The model under review builds one solid part; all positions refer to its coordinate system, in mm. Face numbers are marked on the shaded views. A direction names the side the tool comes from. Coordinates: 2 decimals unless noted, no trailing zeros. Write each loop counter-clockwise with the first axis right and the second up, starting at its lowest first coordinate (ties: lowest second). Pieces come first, ordered by that corner, then holes. Notation, with made-up numbers: (-3.5, 72.5) - (3.5, 72.5) arc R31 ccw to (3.5, 110.5) - close; hole circle Ø11 at (29, 18). An arc over 180 degrees is marked (long way). Return JSON: item names as keys, results as strings. Group by question number.
(1) We need section B-B on z = 21.25. State the section outline as (x, y) points, then the cut area to 3 significant figures.
(2) Tool access review of the marked faces 1, 2 and 3: name each direction out of +Z, -Z, +X, -X, +Y, -Y from which nothing blocks a thin tool from reaching the whole face with its end or side.
(3) For pin 1 Ø5 at (x, z) = (68.18, 6.66) entering from +Y; pin 2 Ø12 at (x, z) = (44.5, 17) entering from +Y; pin 3 Ø3 at (y, z) = (25.5, 7) entering from +X; pin 4 Ø3 at (x, z) = (50.82, 17.34) entering from +Y, all flat-tipped, find the tip position at first contact; note any pin that passes through.
(4) We need section C-C on y = 15.5. State the section outline as (x, z) points.
(5) To check wall thickness, follow L1, parallel to Y at x = 37, z = 20; L2, parallel to Z at x = 20, y = 3.95; L3, parallel to Y at x = 52.5, z = 8.75. State the ranges of each line that lie inside material, in increasing order. Write a range as from..to.
(6) We need section A-A on x = 20. State the section outline as (y, z) points.
(7) Draft analysis for pull direction Y (two halves, no side actions). For the marked faces 4, 5, 6 and 7, state which applies: released by +Y, released by -Y, zero draft, split by the parting line, or undercut.
```python
from build123d import *

# Parameters (mm, degrees)
F0_W      = 40
F0_H      = 6
F0_W_2    = 80
F1_DEPTH  = 24
F2_R      = 1
F3_R      = 1
F4_R      = 1
F5_R      = 1
F6_R      = 1
F7_R      = 1
F8_R      = 1
F10_DEPTH = 6
F11_R     = 2
F12_DEPTH = 6


with BuildPart() as f1:
    # F0 (on Top) → F1 (new body)
    with BuildSketch(Plane.XY):
        with Locations((20, 29)):
            Rectangle(F0_W, F0_H)
        with Locations((40, 3)):
            Rectangle(F0_W_2, F0_H)
        Polygon((-6, 0), (0, 0), (0, 6), (0, 26), (0, 32), (-6, 32), align=None)
    extrude(amount=F1_DEPTH)

    # F2
    f2_edges = [f1.edges().sort_by_distance(p)[0] for p in [
        (0, 6, 12),
    ]]
    fillet(f2_edges, radius=F2_R)

    # F3
    f3_edges = [f1.edges().sort_by_distance(p)[0] for p in [
        (80, 6, 12),
    ]]
    fillet(f3_edges, radius=F3_R)

    # F4
    f4_edges = [f1.edges().sort_by_distance(p)[0] for p in [
        (80, 0, 12),
    ]]
    fillet(f4_edges, radius=F4_R)

    # F5
    f5_edges = [f1.edges().sort_by_distance(p)[0] for p in [
        (0, 26, 12),
    ]]
    fillet(f5_edges, radius=F5_R)

    # F6
    f6_edges = [f1.edges().sort_by_distance(p)[0] for p in [
        (40, 32, 12),
    ]]
    fillet(f6_edges, radius=F6_R)

    # F7
    f7_edges = [f1.edges().sort_by_distance(p)[0] for p in [
        (40, 26, 12),
    ]]
    fillet(f7_edges, radius=F7_R)

    # F8
    f8_edges = [f1.edges().sort_by_distance(p)[0] for p in [
        (-6, 32, 12),
    ]]
    fillet(f8_edges, radius=F8_R)

    # F9 (on face) → F10 (cut)
    with BuildSketch(Plane(origin=(0, 32, 0), x_dir=(-1, 0, 0), z_dir=(0, 1, 0))):
        with BuildLine():
            ThreePointArc((-28, 6), (-23.7573593129, 7.7573593129), (-22, 12))
            ThreePointArc((-22, 12), (-23.7573593129, 16.2426406871), (-28, 18))
            Line((-28, 18), (-28, 6))
        make_face()
        with BuildLine():
            ThreePointArc((-28, 18), (-23.7573593129, 16.2426406871), (-22, 12))
            ThreePointArc((-22, 12), (-23.7573593129, 7.7573593129), (-28, 6))
            Line((-28, 6), (-12, 6))
            ThreePointArc((-12, 6), (-18, 12), (-12, 18))
            Line((-12, 18), (-28, 18))
        make_face()
        with BuildLine():
            Line((-28, 6), (-28, 18))
            ThreePointArc((-28, 18), (-34, 12), (-28, 6))
        make_face()
        with BuildLine():
            Line((-12, 6), (-12, 18))
            ThreePointArc((-12, 18), (-18, 12), (-12, 6))
        make_face()
        with BuildLine():
            ThreePointArc((-6, 12), (-7.7573593129, 16.2426406871), (-12, 18))
            Line((-12, 18), (-12, 6))
            ThreePointArc((-12, 6), (-7.7573593129, 7.7573593129), (-6, 12))
        make_face()
    extrude(amount=-F10_DEPTH, mode=Mode.SUBTRACT)

    # F11 (on face) → F12 (cut)
    with BuildSketch(Plane(origin=(0, 6, 0), x_dir=(-1, 0, 0), z_dir=(0, 1, 0))):
        with Locations((-20, 12)):
            Circle(F11_R)
        with Locations((-68.1839393779, 6.6560373059)):
            Circle(F11_R)
        with Locations((-50.8160606221, 17.3439626941)):
            Circle(F11_R)
    extrude(amount=-F12_DEPTH, mode=Mode.SUBTRACT)


solid = f1.part
```
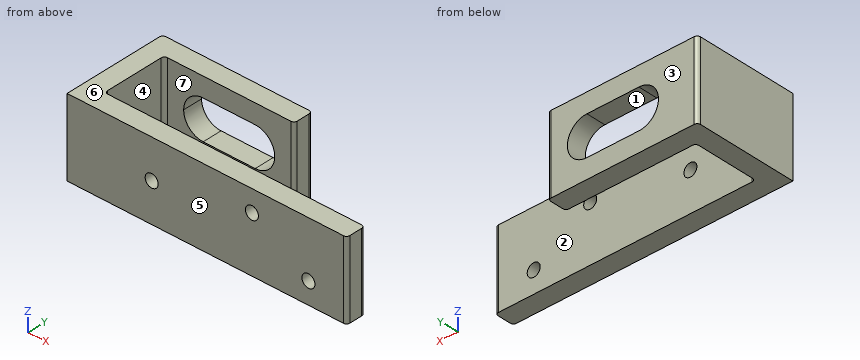
Ans:
{
 "1": {"outline": "(-6, 0) - (79, 0) arc R1 ccw to (80, 1) - (80, 5) arc R1 ccw to (79, 6) - (1, 6) arc R1 cw to (0, 7) - (0, 25) arc R1 cw to (1, 26) - (39, 26) arc R1 ccw to (40, 27) - (40, 31) arc R1 ccw to (39, 32) - (-5, 32) arc R1 ccw to (-6, 31) - close", "area": "911 mm²"},
 "2": {"face 1": "+Y", "face 2": "+Z, -Z, +X", "face 3": "+Z, -Z, +X, -X, +Y"},
 "3": {"pin 1": "y = 6", "pin 2": "y = 32", "pin 3": "x = 40", "pin 4": "through"},
 "4": {"outline": "(-6, 0) - (0, 0) - (0, 24) - (-6, 24) - close"},
 "5": {"L1": "0..6, 26..32", "L2": "0..10, 14..24", "L3": "0..6"},
 "6": {"outline": "(0, 0) - (6, 0) - (6, 10) - (0, 10) - close; (0, 14) - (6, 14) - (6, 24) - (0, 24) - close; (26, 0) - (32, 0) - (32, 6) - (26, 6) - close; (26, 18) - (32, 18) - (32, 24) - (26, 24) - close"},
 "7": {"face 4": "undercut", "face 5": "released by -Y", "face 6": "zero draft", "face 7": "undercut"}
}
